The listing builds one solid part. Answer for the finished solid, in the listing's coordinates (mm). Face numbers are marked on the shaded views. A direction names the side the tool comes from. Give positions to 0.01 mm unless a question says otherwise; leave off trailing zeros. Order: outer loops, then holes, each group sorted by start corner. A loop starts at its lowest first (then second) coordinate and runs counter-clockwise, first axis right, second up. Notation, with made-up numbers: (20, 46.25) - (71, 46.25) arc R24 ccw to (71, 85.25) - close; hole circle Ø7 at (5, 6.25). An arc over 180 degrees is marked (long way). Answer as a JSON object with one key per item and string values. Group by question number.
Q1. For the marked faces 4 and 5, determine the directions among +Z, -Z, +X, -X, +Y, -Y from which every point of the face is accessible in a straight line to the end or side of a thin tool.
Q2. Consider line 1 (Y direction, x = 0, z = 4.5); line 2 (X direction, y = -4, z = 1); line 3 (Y direction, x = 9.25, z = 8.25). Determine where each line is inside the solid, lowest interval first.
Q3. A cutting plane is placed at D-D, the plane z = 4.5. Give the vertices of the cut face in (x, y).
Q4. A cutting plane is placed at A-A, the plane x = 7.75. Give the vertices of the cut face in (y, z).
Q5. A cutting plane is placed at B-B, the plane y = 4. Give the vertices of the cut face in (x, z).
Q6. The mould has two halves that part along X. Classify the marked faces 1, 2 and 3: released by +X, released by -X, zero draft, split by the parting line, or undercut.
Q7. Given pin 1 (3 mm diameter, centred on x = -7, z = 3.5, fed in from +Y); pin 2 (0.8 mm diameter, centred on x = 1.5, z = 10.5, fed in from -Y); pin 3 (5 mm diameter, centred on x = -10.5, z = 6, fed in from -Y); pin 4 (7.5 mm diameter, centred on x = 4, y = 18.5, fed in from +Z), each flat-ended and moving along its own axis, determine where each tip first touches the part or whether it passes through.
Q8. A cutting plane is placed at C-C, the plane x = 0. Give the vertices of the cut face in (y, z).
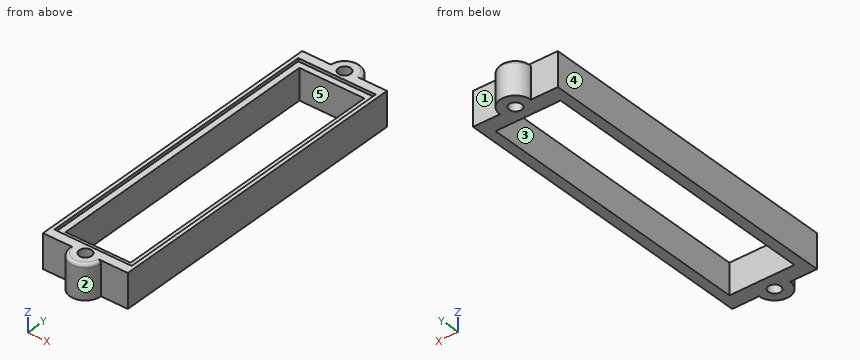
from build123d import *

# Parameters (mm, degrees)
F0_W     = 25
F0_H     = 96.4
F0_W_2   = 21
F0_H_2   = 92.4
F1_DEPTH = 10
F2_DEPTH = 11
F3_D     = 4
F3_DEPTH = 15
F4_R     = 1


with BuildPart() as f1:
    # F0 (on Top) → F1 (new body)
    with BuildSketch(Plane.XY):
        Rectangle(F0_W, F0_H)
        Rectangle(F0_W_2, F0_H_2, mode=Mode.SUBTRACT)
    extrude(amount=F1_DEPTH)

    # F0 (on Top) → F2 (join)
    with BuildSketch(Plane.XY):
        Polygon((-5, 51.2), (-13.7, 51.2), (-13.7, -51.2), (-5, -51.2), (5, -51.2), (13.7, -51.2), (13.7, 51.2), (5, 51.2), align=None)
        Rectangle(F0_W, F0_H, mode=Mode.SUBTRACT)
        with BuildLine():
            Line((5, -51.2), (-5, -51.2))
            ThreePointArc((-5, -51.2), (0, -56.2), (5, -51.2))
        make_face()
        with BuildLine():
            ThreePointArc((5, 51.2), (0, 56.2), (-5, 51.2))
            Line((-5, 51.2), (5, 51.2))
        make_face()
    extrude(amount=F2_DEPTH)

    # F3
    with Locations(Plane(origin=(0, 0, 0), x_dir=(1, 0, 0), z_dir=(0, 0, -1))):
        with Locations((0, 51.2), (0, -51.2)):
            Hole(F3_D / 2, depth=F3_DEPTH)

    # F4
    f4_edges = [f1.edges().sort_by_distance(p)[0] for p in [
        (0, 56.2, 11),
        (0, -56.2, 11),
    ]]
    fillet(f4_edges, radius=F4_R)


solid = f1.part
Reply:
{
 "1": {"face 4": "+Z, -Z, -X, +Y, -Y", "face 5": "+Z, -Z"},
 "2": {"line 1": "y = -56.2 to -53.2, -49.2 to -46.2, 46.2 to 49.2, 53.2 to 56.2", "line 2": "x = -13.7 to -10.5, 10.5 to 13.7", "line 3": "y = -51.2 to -46.2, 46.2 to 51.2"},
 "3": {"outline": "(-13.7, -51.2) - (-5, -51.2) arc R5 ccw to (5, -51.2) - (13.7, -51.2) - (13.7, 51.2) - (5, 51.2) arc R5 ccw to (-5, 51.2) - (-13.7, 51.2) - close; hole (-10.5, -46.2) - (10.5, -46.2) - (10.5, 46.2) - (-10.5, 46.2) - close; hole circle Ø4 at (0, -51.2); hole circle Ø4 at (0, 51.2)"},
 "4": {"outline": "(-51.2, 0) - (-46.2, 0) - (-46.2, 10) - (-48.2, 10) - (-48.2, 11) - (-51.2, 11) - close; (46.2, 0) - (51.2, 0) - (51.2, 11) - (48.2, 11) - (48.2, 10) - (46.2, 10) - close"},
 "5": {"outline": "(-13.7, 0) - (-10.5, 0) - (-10.5, 10) - (-12.5, 10) - (-12.5, 11) - (-13.7, 11) - close; (10.5, 0) - (13.7, 0) - (13.7, 11) - (12.5, 11) - (12.5, 10) - (10.5, 10) - close"},
 "6": {"face 1": "zero draft", "face 2": "split by the parting line", "face 3": "undercut"},
 "7": {"pin 1": "stops at y = 51.2", "pin 2": "stops at y = -56.03", "pin 3": "stops at y = -51.2", "pin 4": "passes through"},
 "8": {"outline": "(-56.2, 0) - (-53.2, 0) - (-53.2, 11) - (-55.2, 11) arc R1 ccw to (-56.2, 10) - close; (-49.2, 0) - (-46.2, 0) - (-46.2, 10) - (-48.2, 10) - (-48.2, 11) - (-49.2, 11) - close; (46.2, 0) - (49.2, 0) - (49.2, 11) - (48.2, 11) - (48.2, 10) - (46.2, 10) - close; (53.2, 0) - (56.2, 0) - (56.2, 10) arc R1 ccw to (55.2, 11) - (53.2, 11) - close"}
}
